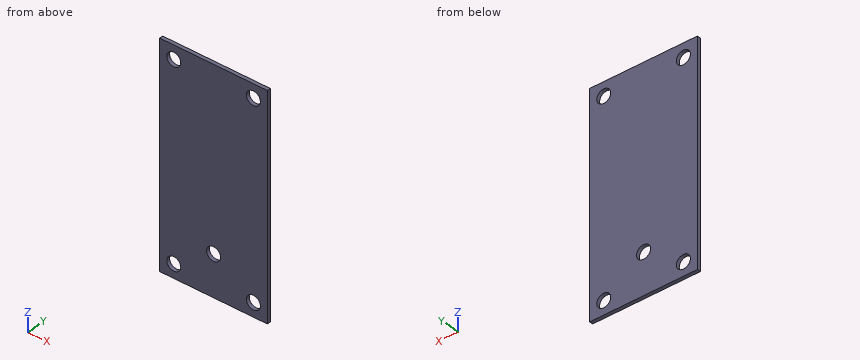
```python
from build123d import *

# Parameters (mm, degrees)
SKETCH1_W           = 48.768
SKETCH1_H           = 101.6
SKETCH1_R           = 3.175
BOSS_EXTRUDE1_DEPTH = 1.5875
CUT_EXTRUDE1_REACH  = 3.587
SKETCH2_R           = 3.175


with BuildPart() as part:
    # Sketch1 → Boss-Extrude1 (new body)
    with BuildSketch(Plane(origin=(0, 0, 0), x_dir=(1, 0, 0), z_dir=(0, 1, 0))):
        Rectangle(SKETCH1_W, SKETCH1_H)
        with Locations((-18.034, 44.45)):
            Circle(SKETCH1_R, mode=Mode.SUBTRACT)
        with Locations((18.034, 44.45)):
            Circle(SKETCH1_R, mode=Mode.SUBTRACT)
        with Locations((18.034, -44.45)):
            Circle(SKETCH1_R, mode=Mode.SUBTRACT)
        with Locations((-18.034, -44.45)):
            Circle(SKETCH1_R, mode=Mode.SUBTRACT)
    extrude(amount=BOSS_EXTRUDE1_DEPTH)

    # Sketch2 → Cut-Extrude1 (cut, up to next)
    with BuildSketch(Plane(origin=(0, 1.5875, 0), x_dir=(1, 0, 0), z_dir=(0, 1, 0)), mode=Mode.PRIVATE) as cut_extrude1_sk1:
        with Locations((0, 31.75)):
            Circle(SKETCH2_R)
    cut_extrude1_tool1 = extrude(cut_extrude1_sk1.sketch, amount=-CUT_EXTRUDE1_REACH, mode=Mode.PRIVATE) & part.part
    add(cut_extrude1_tool1.solids().sort_by_distance((0, 1.5875, -31.75))[0], mode=Mode.SUBTRACT)


solid = part.part
```
Can you work these out from the model? Positions are in its coordinate system, mm. Round coordinates to 2 decimals unless told otherwise and drop trailing zeros. Loops run counter-clockwise (first coordinate to the right, second up) from the corner with the lowest first, then second, coordinate; pieces in that order, holes last. Notation, with made-up numbers: (-14, 19.25) -> (23, 19.25) arc R30 ccw to (23, 42.25) -> close; hole circle Ø8 at (13, 28). An arc over 180 degrees is marked (long way). Answer in a Markdown table with one row per item.
Item 1: Suppose I cut it at B-B, the plane z = -44.45. List the corners of the cut face in (x, y) for me, plus the area to 3 significant figures.
Answer block:
| item | result |
|---|---|
| outline | (-24.38, 0) -> (-21.21, 0) -> (-21.21, 1.59) -> (-24.38, 1.59) -> close; (-14.86, 0) -> (14.86, 0) -> (14.86, 1.59) -> (-14.86, 1.59) -> close; (21.21, 0) -> (24.38, 0) -> (24.38, 1.59) -> (21.21, 1.59) -> close |
| area | 57.3 mm² |
Item 2: Suppose I cut it at D-D, the plane x = 0. List the corners of the cut face in (y, z) for me (1 decimal).
Answer block:
| item | result |
|---|---|
| outline | (0, -50.8) -> (1.6, -50.8) -> (1.6, -34.9) -> (0, -34.9) -> close; (0, -28.6) -> (1.6, -28.6) -> (1.6, 50.8) -> (0, 50.8) -> close |
Item 3: Suppose I cut it at A-A, the plane z = -31.75. List the corners of the cut face in (x, y) for me (1 decimal), plus the area to 3 significant figures.
Answer block:
| item | result |
|---|---|
| outline | (-24.4, 0) -> (-3.2, 0) -> (-3.2, 1.6) -> (-24.4, 1.6) -> close; (3.2, 0) -> (24.4, 0) -> (24.4, 1.6) -> (3.2, 1.6) -> close |
| area | 67.3 mm² |
Item 4: If I drill on probe 1 along X at (y, z) = (1.25, 44.45); probe 2 along X at (y, z) = (1, -31.5); probe 3 along Z at (x, y) = (-20, 1.2), over which ranges is the centre line in solid material (lowest first)?
Answer block:
| item | result |
|---|---|
| probe 1 | -24.38 to -21.21, -14.86 to 14.86, 21.21 to 24.38 |
| probe 2 | -24.38 to -3.17, 3.17 to 24.38 |
| probe 3 | -50.8 to -46.94, -41.96 to 41.96, 46.94 to 50.8 |
Item 5: Suppose I cut it at C-C, the plane x = -19. List the corners of the cut face in (y, z) for me, plus the area to 3 significant figures.
Answer block:
| item | result |
|---|---|
| outline | (0, -50.8) -> (1.59, -50.8) -> (1.59, -47.47) -> (0, -47.47) -> close; (0, -41.43) -> (1.59, -41.43) -> (1.59, 41.43) -> (0, 41.43) -> close; (0, 47.47) -> (1.59, 47.47) -> (1.59, 50.8) -> (0, 50.8) -> close |
| area | 142 mm² |
